Can you work these out from the drawing? Everything is in mm from the part's minimum corner. A direction names the side the tool comes from. Give positions to 0.01 mm unless a question says otherwise; leave off trailing zeros. Write each loop counter-clockwise with the first axis right and the second up, starting at its lowest first coordinate (ties: lowest second). Pieces come first, ordered by that corner, then holes. Notation, with made-up numbers: (17.5, -36) - (31.5, -36) arc R22 ccw to (31.5, -1) - close; hole circle Ø5 at (36, 61). An arc over 180 degrees is marked (long way). Write each question's results on one line, items separated by ' | '. Start each with the question number.
Item 1: Will these pins go through, and if not, where does the flat tip stop? P1, Ø1.9, axis at x = 4.76, y = 19.05, coming from the +Z side; P2, Ø5, axis at x = 41.5, y = 13.5, coming from the +Z side; P3, Ø2.5, axis at x = 71.44, y = 57.15, coming from the -Z side.
Item 2: We'd pull the mould along X, two halves only. Please class the marked faces 3, 4, 5 and 6: +X half, -X half, draft (parallel to the pull), parting line (faces both ways), or undercut.
Item 3: Which directions (+Z, -Z, +X, -X, +Y, -Y) give clear straight access to the entire face, cutting with the end or side of a thin tool? Please do the marked faces 1 and 2.
Item 4: Suppose I cut it at A-A on x = 54. List the corners of the cut face in (y, z) for me (1 decimal).
Item 5: Suppose I cut it at D-D on y = 6.5. List the corners of the cut face in (x, z) for me.
Item 6: Please list where these lines run through material, in increasing order: line 1 along X through (y, z) = (38, 109) (1 decimal); line 2 along X through (y, z) = (13.5, 130.5) (1 decimal).
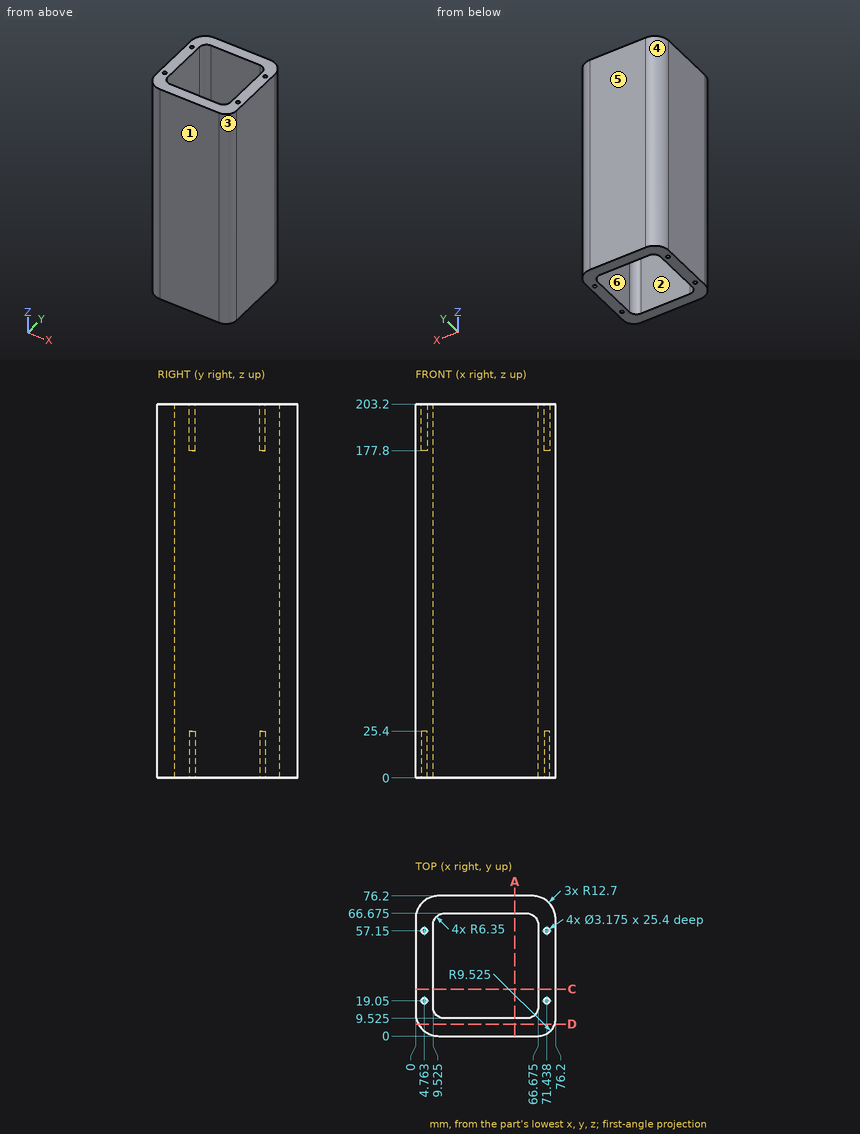
Checked values:
1) P1: stops at z = 177.8 | P2: passes through | P3: stops at z = 25.4
2) face 3: +X half | face 4: -X half | face 5: draft | face 6: undercut
3) face 1: +Z, -Z, +X, -X, -Y | face 2: +Z, -Z
4) outline: (0, 0) - (9.5, 0) - (9.5, 203.2) - (0, 203.2) - close; (66.7, 0) - (76.2, 0) - (76.2, 203.2) - (66.7, 203.2) - close
5) outline: (1.62, 0) - (75.71, 0) - (75.71, 203.2) - (1.62, 203.2) - close
6) line 1: x = 0 to 9.5, 66.7 to 76.2 | line 2: x = 0 to 10, 66.2 to 76.2
